Here's how the part is built. I have some questions about the finished solid (model axes, mm). A direction names the side the tool comes from. Coordinates: 2 decimals unless noted, no trailing zeros. Order: outer loops, then holes, each group sorted by start corner. A loop starts at its lowest first (then second) coordinate and runs counter-clockwise, first axis right, second up. Notation, with made-up numbers: (57.25, 60) - (82.25, 60) arc R30 ccw to (82.25, 89) - close; hole circle Ø5 at (-9, 7.5). An arc over 180 degrees is marked (long way). Answer in a Markdown table with one row per item. Add a question column.
Item 1: Thinking about a two-plate mould opening in Y: for faces 3 (the cylindrical face through (-1.86, 14.18, -1.3)), 4 (the flat face through (-7, -13, -92.5)), 5 (the cylindrical face through (-13.887, -10.648, -87.43)), which applies, +Y half, -Y half, draft (parallel to the pull), parting line (faces both ways), or undercut?
Item 2: Will these pins go through, and if not, where does the flat tip stop? pin 1 Ø12 at (y, z) = (10, 48.5) entering from +X; pin 2 Ø4 at (x, z) = (-7.5, -55) entering from +Y; pin 3 Ø8 at (x, z) = (-8.5, 50) entering from -Y.
Item 3: I want a section at C-C (z = -67.5). Please give me the cut outline in (x, y), plus the area to 3 significant figures.
Item 4: If I drill on line 1 along Y through (x, z) = (0, -32); line 2 along Y through (x, z) = (9.5, -38.5); line 3 along X through (y, z) = (1.5, -83), over which ranges is the centre line in solid material (lowest first)? Write a range as from..to.
Item 5: On a 3-axis mill with a long thin cutter (end or side, diameter ignored), from which of +Z, -Z, +X, -X, +Y, -Y can I reach the whole of each face in a straight line? I mean faces 1 (the cylindrical face through (-13.887, -10.648, 87.57)), 2 (the flat face through (0, -17, 82.5)). Say none if no direction works.
Item 6: I want a section at A-A (x = 0). Please give me the cut outline in (y, z), plus the area to 4 significant figures.
```python
from build123d import *

# Parameters (mm, degrees)
ESQUISSE1_R             = 17.5
ESQUISSE1_R_2           = 14.3
BOSS_EXTRU_1_DEPTH      = 92.5
ESQUISSE2_OUTSIDE_W     = 75.302
ESQUISSE2_OUTSIDE_H     = 75.302
ESQUISSE2_OUTSIDE_R     = 16.75
ENL_V_MAT_EXTRU_1_DEPTH = 82.5


with BuildPart() as part:
    # Esquisse1 → Boss.-Extru.1 (new, symmetric)
    with BuildSketch(Plane.XY):
        Circle(ESQUISSE1_R)
        Circle(ESQUISSE1_R_2, mode=Mode.SUBTRACT)
    extrude(amount=BOSS_EXTRU_1_DEPTH, both=True)

    # Esquisse2 outside → Enlèv. mat.-Extru.1 (cut, symmetric)
    with BuildSketch(Plane.XY):
        Rectangle(ESQUISSE2_OUTSIDE_W, ESQUISSE2_OUTSIDE_H)
        Circle(ESQUISSE2_OUTSIDE_R, mode=Mode.SUBTRACT)
    extrude(amount=ENL_V_MAT_EXTRU_1_DEPTH, both=True, mode=Mode.SUBTRACT)


solid = part.part
```
Values follow:
| question | item | result |
|---|---|---|
| 1 | face 3 | undercut |
| 1 | face 4 | draft |
| 1 | face 5 | parting line |
| 2 | pin 1 | stops at x = 16.27 |
| 2 | pin 2 | stops at y = 15.82 |
| 2 | pin 3 | stops at y = -16.13 |
| 3 | outline | circle Ø33.5 at (0, 0); hole circle Ø28.6 at (0, 0) |
| 3 | area | 239 mm^2 |
| 4 | line 1 | y = -16.75..-14.3, 14.3..16.75 |
| 4 | line 2 | y = -13.8..-10.69, 10.69..13.8 |
| 4 | line 3 | x = -17.44..-14.22, 14.22..17.44 |
| 5 | face 1 | +Z, -Z |
| 5 | face 2 | none |
| 6 | outline | (-17.5, -92.5) - (-14.3, -92.5) - (-14.3, 92.5) - (-17.5, 92.5) - (-17.5, 82.5) - (-16.75, 82.5) - (-16.75, -82.5) - (-17.5, -82.5) - close; (14.3, -92.5) - (17.5, -92.5) - (17.5, -82.5) - (16.75, -82.5) - (16.75, 82.5) - (17.5, 82.5) - (17.5, 92.5) - (14.3, 92.5) - close |
| 6 | area | 936.5 mm^2 |
